Can you work these out from the drawing? Everything is in mm from the part's minimum corner. Round coordinates to 2 decimals unless told otherwise and drop trailing zeros. Loops run counter-clockwise (first coordinate to the right, second up) from the corner with the lowest first, then second, coordinate; pieces in that order, holes last. Notation, with made-up numbers: M -24,79 L 4,79 A18 ccw 4,114 Z; hole C -24.75,-8.75 d1. An arc over 180 degrees is marked long. Answer in a Markdown table with one row per item.
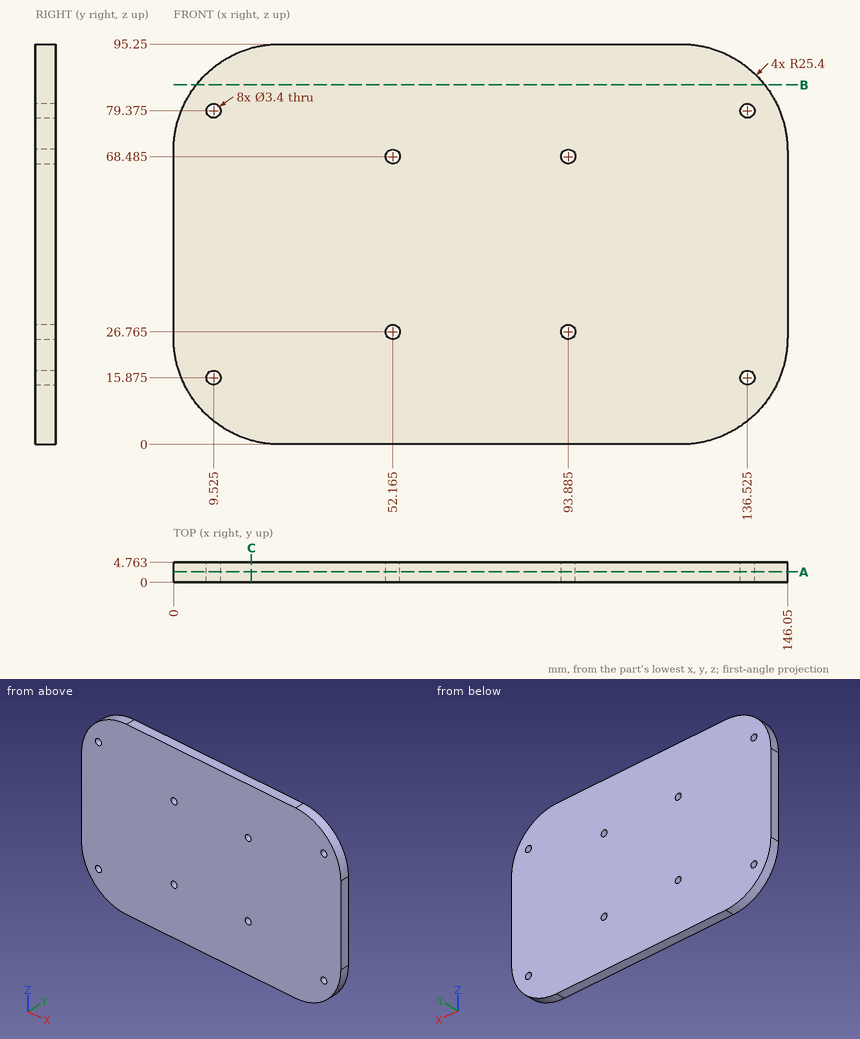
1) I want a section at A-A, the plane y = 2.5. State how many separate pieces and enclosed holes the cut face has, plus the area to 3 significant figures.
Computed:
| item | result |
|---|---|
| separate pieces | 1 |
| enclosed holes | 8 |
| area | 13,300 mm² |
2) Will this pin go through, and if not, where does the flat tip stop? P1, Ø1, axis at y = 1, z = 84.5, coming from the -X side (1 decimal).
Computed:
| item | result |
|---|---|
| P1 | stops at x = 4.3 |
3) I need wall thicknesses on line 1 (Z direction, x = 52, y = 1.5); line 2 (X direction, y = 0.4, z = 25); line 3 (Z direction, x = 25, y = 3.75). Which ranges of each line are inside material? Lowest first, please.
Computed:
| item | result |
|---|---|
| line 1 | z = 0 to 25.07, 28.46 to 66.79, 70.18 to 95.25 |
| line 2 | x = 0 to 146.05 |
| line 3 | z = 0 to 95.25 |
4) I want a section at C-C, the plane x = 18.5. Please give me the cut outline in (y, z) (1 decimal).
Computed:
| item | result |
|---|---|
| outline | M 0,1 L 4.8,1 L 4.8,94.3 L 0,94.3 Z |
5) I want a section at B-B, the plane z = 85.5. Please give me the cut outline in (x, y) (1 decimal).
Computed:
| item | result |
|---|---|
| outline | M 5.4,0 L 140.7,0 L 140.7,4.8 L 5.4,4.8 Z |
